from build123d import *

# Parameters (mm, degrees)
SKETCH1_R           = 5
BOSS_EXTRUDE1_DEPTH = 45
SKETCH4_R           = 1.5
CUT_EXTRUDE1_DEPTH  = 46.552167896


with BuildPart() as part:
    # Sketch1 → Boss-Extrude1 (new, symmetric)
    with BuildSketch(Plane(origin=(0, 0, 0), x_dir=(0, 0, -1), z_dir=(1, 0, 0))):
        with Locations(Location((0, 0, 0), (0, 0, 180))):
            Circle(SKETCH1_R)
    extrude(amount=BOSS_EXTRUDE1_DEPTH, both=True)

    # Sketch4 → Cut-Extrude1 (cut, symmetric)
    with BuildSketch(Plane(origin=(0, 0, 0), x_dir=(1, 0, 0), z_dir=(0, 1, 0))):
        with Locations(Location((-40, 0, 0), (0, 0, 270))):
            Circle(SKETCH4_R)
    cut_extrude1 = extrude(amount=CUT_EXTRUDE1_DEPTH, both=True, mode=Mode.SUBTRACT)

    # Mirror1: Cut-Extrude1 across plane
    add(cut_extrude1.mirror(Plane(origin=(0, 0, 0), x_dir=(0, 0, 1), z_dir=(1, 0, 0))), mode=Mode.SUBTRACT)


solid = part.part
Geometry: final body of the model. Coordinates: model frame, mm. Give positions to 0.01 mm unless a question says otherwise; leave off trailing zeros. Loops run counter-clockwise (first coordinate to the right, second up) from the corner with the lowest first, then second, coordinate; pieces in that order, holes last. Notation, with made-up numbers: M 61.25,-12 L 110.25,-12 A12 ccw 110.25,9 Z; hole C 43.5,46.5 d1. An arc over 180 degrees is marked long. Put each result on its own line as item: value. Start each with the question number.
1) Cut plane D-D (z = 4). Output: boundary loops of the cut face in (x, y), then the cut area to 3 significant figures.
2) Cut plane B-B (z = -0.5). Output: boundary loops of the cut face in (x, y).
3) Pull-direction query (Z, two-part tool) for faces 1 (the cylindrical face through (0.63, -1.5, 4.77)), 2 (the cylindrical face through (-41.464, 0.07, -0.325)), 3 (the flat face through (45, 0, 0)); classes: pulls with the +Z half, pulls with the -Z half, needs draft (parallel to the pull), parting line crosses it, or undercut.
4) Ray query, line 1 along X through (y, z) = (1.25, 0); line 2 along X through (y, z) = (1.25, -1); line 3 along Z through (x, y) = (-40, -2.25). Return the intervals inside material, ascending.
5) Cut plane C-C (x = 16.5). Output: boundary loops of the cut face in (y, z), then the cut area to 3 significant figures.
6) Contact query for flat-ended pins moving along their axis: pin 1 (3 mm diameter, centred on x = -27.5, y = 1.5, fed in from -Z); pin 2 (1.5 mm diameter, centred on x = -4.5, y = -4, fed in from -Z); pin 3 (2 mm diameter, centred on x = -24.5, y = 2.5, fed in from +Z); pin 4 (3 mm diameter, centred on x = -9, z = 2, fed in from -Y). Output: stop coordinate, or through.
7) Cut plane A-A (y = 0). Output: boundary loops of the cut face in (x, z).
Verdict:
1. outline: M -45,-3 L 45,-3 L 45,3 L -45,3 Z
1. area: 540 mm2
2. outline: M -45,-4.97 L -41.41,-4.97 L -41.41,4.97 L -45,4.97 Z; M -38.59,-4.97 L 38.59,-4.97 L 38.59,4.97 L -38.59,4.97 Z; M 41.41,-4.97 L 45,-4.97 L 45,4.97 L 41.41,4.97 Z
3. face 1: parting line crosses it
3. face 2: undercut
3. face 3: needs draft
4. line 1: -45 to -41.5, -38.5 to 38.5, 41.5 to 45
4. line 2: -45 to -41.12, -38.88 to 38.88, 41.12 to 45
4. line 3: -4.47 to -1.5, 1.5 to 4.47
5. outline: C 0,0 d10
5. area: 78.5 mm2
6. pin 1: z = -5
6. pin 2: z = -3.8
6. pin 3: z = 4.77
6. pin 4: y = -4.97
7. outline: M -45,-5 L 45,-5 L 45,5 L -45,5 Z; hole C -40,0 d3; hole C 40,0 d3
